Could you check a few things on this model? Use its own coordinates, in mm. A direction names the side the tool comes from. Coordinates: 2 decimals unless noted, no trailing zeros. Order: outer loops, then holes, each group sorted by start corner. A loop starts at its lowest first (then second) coordinate and runs counter-clockwise, first axis right, second up. Notation, with made-up numbers: (85.25, 14.25) -> (127.25, 14.25) arc R28 cw to (127.25, 45.25) -> close; hole circle Ø2 at (48.5, -36.75). An arc over 180 degrees is marked (long way). Use a Markdown table: item, result. Add a question column.
1) If we section it at C-C (y = 55.5): Write out the boundary of the cut face in (x, z), plus the area to 3 significant figures.
2) If we section it at A-A (x = 8.05): Give the number of separate pieces and of enclosed holes in the cut face, plus the area to 3 significant figures.
3) Which directions (+Z, -Z, +X, -X, +Y, -Y) give clear straight access to the entire face, cutting with the end or side of a thin tool? Please do faces 4 (the flat face through (-62, 27, 18)), 5 (the flat face through (74, 10, 99)), 6 (the flat face through (-55, 36, 9)), 7 (the flat face through (63, 14, 110)).
4) If I drill on L1, parallel to X at y = 6.75, z = 101; L2, parallel to Z at x = 8.05, y = 73.65; L3, parallel to Y at x = -46, z = 90, over which ranges is the centre line in solid material (lowest first)? Write a range as [from, to].
5) If we section it at D-D (x = -77): Write out the boundary of the cut face in (y, z).
6) If we section it at B-B (z = 55): Write out the boundary of the cut face in (x, y).
7) Will these pins go through, and if not, where does the flat tip stop? pin 1 Ø21.5 at (x, y) = (-72, 22.5) entering from +Z; pin 2 Ø2 at (x, z) = (-67, 99) entering from +Y; pin 3 Ø5 at (y, z) = (35, 15.5) entering from +X; pin 4 Ø8.5 at (x, z) = (77, 9) entering from -Y.
8) Thinking about a two-plate mould opening in X: for faces 1 (the flat face through (-55, 36, 101)), 2 (the flat face through (85, 5, 101)), 3 (the flat face through (1, 41, 113)), which applies, +X half, -X half, draft (parallel to the pull), parting line (faces both ways), or undercut?
```python
from build123d import *

# Parameters (mm, degrees)
BOSS_EXTRUDE2_DEPTH = 110
SKETCH4_W           = 74
SKETCH4_H           = 70.5
CUT_EXTRUDE2_DEPTH  = 218.899632859
CUT_EXTRUDE3_REACH  = 162.64
SKETCH5_R           = 40
CUT_EXTRUDE4_REACH  = 157.869
SKETCH6_R           = 3.25
SKETCH7_W           = 130
SKETCH7_H           = 10
BOSS_EXTRUDE3_DEPTH = 3
CHAMFER1_SIZE       = 3
CHAMFER2_SIZE       = 5
CHAMFER3_SIZE       = 3
CHAMFER5_SIZE       = 3


# Some blends are built 0.0001 mm under size
with BuildPart() as part:
    # Sketch3 → Boss-Extrude2 (new body)
    with BuildSketch(Plane.XY):
        Polygon((65, 10), (85, 10), (85, 0), (55, 0), (55, 70.5), (-55, 70.5), (-55, 0), (-85, 0), (-85, 10), (-65, 10), (-65, 80.5), (65, 80.5), align=None)
    extrude(amount=BOSS_EXTRUDE2_DEPTH)

    # Sketch4 → Cut-Extrude2 (cut, through all)
    with BuildSketch(Plane(origin=(85, 0, 0), x_dir=(0, 0, -1), z_dir=(1, 0, 0))):
        with Locations((-55, 35.25)):
            Rectangle(SKETCH4_W, SKETCH4_H)
    extrude(amount=-CUT_EXTRUDE2_DEPTH, mode=Mode.SUBTRACT)

    # Sketch5 → Cut-Extrude3 (cut, up to next)
    with BuildSketch(Plane(origin=(0, 80.5, 0), x_dir=(1, 0, 0), z_dir=(0, 1, 0)), mode=Mode.PRIVATE) as cut_extrude3_sk1:
        with Locations(Location((8.05, -55, 0), (0, 0, 180))):
            Circle(SKETCH5_R)
    cut_extrude3_tool1 = extrude(cut_extrude3_sk1.sketch, amount=-CUT_EXTRUDE3_REACH, mode=Mode.PRIVATE) & part.part
    add(cut_extrude3_tool1.solids().sort_by_distance((8.05, 80.5, 55))[0], mode=Mode.SUBTRACT)

    # Sketch6 → Cut-Extrude4 (cut, up to next)
    with BuildSketch(Plane(origin=(0, 10, 0), x_dir=(1, 0, 0), z_dir=(0, 1, 0)), mode=Mode.PRIVATE) as cut_extrude4_sk1:
        with Locations(Location((77, -101, 0), (0, 0, 270))):
            Circle(SKETCH6_R)
    cut_extrude4_tool1 = extrude(cut_extrude4_sk1.sketch, amount=-CUT_EXTRUDE4_REACH, mode=Mode.PRIVATE) & part.part
    # Sketch6 → Cut-Extrude4 (cut, up to next)
    with BuildSketch(Plane(origin=(0, 10, 0), x_dir=(1, 0, 0), z_dir=(0, 1, 0)), mode=Mode.PRIVATE) as cut_extrude4_sk2:
        with Locations(Location((77, -9, 0), (0, 0, 270))):
            Circle(SKETCH6_R)
    cut_extrude4_tool2 = extrude(cut_extrude4_sk2.sketch, amount=-CUT_EXTRUDE4_REACH, mode=Mode.PRIVATE) & part.part
    # Sketch6 → Cut-Extrude4 (cut, up to next)
    with BuildSketch(Plane(origin=(0, 10, 0), x_dir=(1, 0, 0), z_dir=(0, 1, 0)), mode=Mode.PRIVATE) as cut_extrude4_sk3:
        with Locations(Location((-77, -9, 0), (0, 0, 270))):
            Circle(SKETCH6_R)
    cut_extrude4_tool3 = extrude(cut_extrude4_sk3.sketch, amount=-CUT_EXTRUDE4_REACH, mode=Mode.PRIVATE) & part.part
    # Sketch6 → Cut-Extrude4 (cut, up to next)
    with BuildSketch(Plane(origin=(0, 10, 0), x_dir=(1, 0, 0), z_dir=(0, 1, 0)), mode=Mode.PRIVATE) as cut_extrude4_sk4:
        with Locations(Location((-77, -101, 0), (0, 0, 270))):
            Circle(SKETCH6_R)
    cut_extrude4_tool4 = extrude(cut_extrude4_sk4.sketch, amount=-CUT_EXTRUDE4_REACH, mode=Mode.PRIVATE) & part.part
    add(cut_extrude4_tool1.solids().sort_by_distance((77, 10, 101))[0], mode=Mode.SUBTRACT)
    add(cut_extrude4_tool2.solids().sort_by_distance((77, 10, 9))[0], mode=Mode.SUBTRACT)
    add(cut_extrude4_tool3.solids().sort_by_distance((-77, 10, 9))[0], mode=Mode.SUBTRACT)
    add(cut_extrude4_tool4.solids().sort_by_distance((-77, 10, 101))[0], mode=Mode.SUBTRACT)

    # Sketch7 → Boss-Extrude3 (add)
    with BuildSketch(Plane(origin=(0, 0, 0), x_dir=(-1, 0, 0), z_dir=(0, 0, -1))):
        with Locations((0, 40.5)):
            Rectangle(SKETCH7_W, SKETCH7_H)
    boss_extrude3 = extrude(amount=BOSS_EXTRUDE3_DEPTH)

    # Mirror1: Boss-Extrude3 across plane
    add(boss_extrude3.mirror(Plane.XY.offset(55)))

    # Chamfer1
    chamfer1_edges = [part.edges().sort_by_distance(p)[0] for p in [
        (0, 35.5, -3),
        (0, 45.5, -3),
    ]]
    chamfer(chamfer1_edges, length=CHAMFER1_SIZE - 0.0001)  # a hair under: the kernel refuses the full size

    # Chamfer2
    chamfer2_edges = [part.edges().sort_by_distance(p)[0] for p in [
        (0, 80.5, 0),
        (0, 80.5, 110),
        (-65, 80.5, 55),
        (65, 80.5, 55),
        (48.05, 80.5, 55),
    ]]
    chamfer(chamfer2_edges, length=CHAMFER2_SIZE)

    # Chamfer3
    # the kernel refuses this chamfer: 3 mm, written as the material it takes off along each edge
    with BuildSketch(Plane(origin=(-72.715048964, 35.5, 113), x_dir=(0, 0.9996219169112965, 0.02749587661058676), z_dir=(1, 0, 0))) as chamfer3_piece_1:
        Polygon((CHAMFER3_SIZE * 0.999621916911, -CHAMFER3_SIZE * 0.0274958766106), (-CHAMFER3_SIZE * 0.0274958766106, -CHAMFER3_SIZE * 0.999621916911), (0, 0), align=None)
    extrude(amount=145.430097928, mode=Mode.SUBTRACT)
    with BuildSketch(Plane(origin=(72.715048964, 45.5, 113), x_dir=(0, 0.027495876610586768, -0.9996219169112968), z_dir=(-1, 0, 0))) as chamfer3_piece_2:
        Polygon((CHAMFER3_SIZE * 0.999621916911, CHAMFER3_SIZE * 0.0274958766106), (-CHAMFER3_SIZE * 0.0274958766106, CHAMFER3_SIZE * 0.999621916911), (0, 0), align=None)
    extrude(amount=145.430097928, mode=Mode.SUBTRACT)

    # Chamfer5
    chamfer5_edges = [part.edges().sort_by_distance(p)[0] for p in [
        (-85, 5, 0),
        (85, 5, 0),
        (-65, 10, 101),
        (65, 10, 101),
        (-85, 5, 110),
        (-65, 10, 9),
        (65, 10, 9),
        (85, 5, 18),
        (-85, 5, 92),
        (-85, 5, 18),
        (85, 5, 92),
        (85, 5, 110),
    ]]
    chamfer(chamfer5_edges, length=CHAMFER5_SIZE)


solid = part.part
```
Answer sheet:
| question | item | result |
|---|---|---|
| 1 | outline | (-65, 0) -> (-55, 0) -> (-55, 18) -> (-65, 18) -> close; (-65, 92) -> (-55, 92) -> (-55, 110) -> (-65, 110) -> close; (55, 0) -> (65, 0) -> (65, 18) -> (55, 18) -> close; (55, 92) -> (65, 92) -> (65, 110) -> (55, 110) -> close |
| 1 | area | 720 mm2 |
| 2 | separate pieces | 4 |
| 2 | enclosed holes | 0 |
| 2 | area | 292 mm2 |
| 3 | face 4 | +X, -X, -Y |
| 3 | face 5 | +Z, -Z, +X, +Y |
| 3 | face 6 | -Y |
| 3 | face 7 | +Z, +X, -X, -Y |
| 4 | L1 | [-85, -80.25], [-73.75, -55], [55, 73.75], [80.25, 85] |
| 4 | L2 | [0, 15], [95, 110] |
| 4 | L3 | [70.5, 80.5] |
| 5 | outline | (0, 0) -> (10, 0) -> (10, 5.75) -> (0, 5.75) -> close; (0, 12.25) -> (10, 12.25) -> (10, 18) -> (0, 18) -> close; (0, 92) -> (10, 92) -> (10, 97.75) -> (0, 97.75) -> close; (0, 104.25) -> (10, 104.25) -> (10, 110) -> (0, 110) -> close |
| 6 | outline | (-65, 70.5) -> (-31.95, 70.5) -> (-31.95, 75.5) -> (-36.95, 80.5) -> (-60, 80.5) -> (-65, 75.5) -> close; (48.05, 70.5) -> (65, 70.5) -> (65, 75.5) -> (60, 80.5) -> (53.05, 80.5) -> (48.05, 75.5) -> close |
| 7 | pin 1 | z = 110 |
| 7 | pin 2 | y = 12 |
| 7 | pin 3 | x = 65 |
| 7 | pin 4 | y = 0 |
| 8 | face 1 | undercut |
| 8 | face 2 | +X half |
| 8 | face 3 | draft |
